```python
from build123d import *

# Parameters (mm, degrees)
SKETCH_1_W      = 6
SKETCH_1_H      = 6
EXTRUDE_1_DEPTH = 3.5
SKETCH_2_R      = 1.75
EXTRUDE_2_DEPTH = 5


with BuildPart() as part:
    # 草图1 → 凸台-拉伸1 (new body)
    with BuildSketch(Plane(origin=(0, 0, 0), x_dir=(1, 0, 0), z_dir=(0, 1, 0))):
        Rectangle(SKETCH_1_W, SKETCH_1_H)
    extrude(amount=EXTRUDE_1_DEPTH)

    # 草图2 → 凸台-拉伸2 (add)
    with BuildSketch(Plane.XZ):
        Circle(SKETCH_2_R)
    extrude(amount=-EXTRUDE_2_DEPTH)


solid = part.part
```
Geometry: final body of the model. Coordinates: model frame, mm. A direction names the side the tool comes from. Coordinates: 2 decimals unless noted, no trailing zeros. Order: outer loops, then holes, each group sorted by start corner. A loop starts at its lowest first (then second) coordinate and runs counter-clockwise, first axis right, second up. Notation, with made-up numbers: (-25, -29) -> (12, -29) arc R8 ccw to (12, -18) -> close; hole circle Ø1 at (-18, -3). An arc over 180 degrees is marked (long way). Use CSV: the item, a comma, the result in double quotes.
1) Section C-C on y = 3.7. Output: boundary loops of the cut face in (x, z), then the cut area to 3 significant figures.
Findings:
outline,"circle Ø3.5 at (0, 0)"
area,"9.62 mm^2"
2) Section A-A on z = 0. Output: boundary loops of the cut face in (x, y), then the cut area to 4 significant figures.
Findings:
outline,"(-3, 0) -> (3, 0) -> (3, 3.5) -> (1.75, 3.5) -> (1.75, 5) -> (-1.75, 5) -> (-1.75, 3.5) -> (-3, 3.5) -> close"
area,"26.25 mm^2"
3) Access query for faces 1 (the flat face through (0, 2, -3)), 2 (the flat face through (1.3, 3.5, -1.4)). Directions: +Z, -Z, +X, -X, +Y, -Y. A direction counts if a zero-diameter tool reaches every point of the face in a straight line with its end or side. Return the directions, or none.
Findings:
face 1,"-Z, +X, -X, +Y, -Y"
face 2,"+Y"
4) Line query: line 1 (Y direction, x = -1.3, z = 2); line 2 (Z direction, x = 1.5, y = 4.05); line 3 (X direction, y = 4, z = -0.35). Output: solid intervals per line, ascending.
Findings:
line 1,"y = 0 to 3.5"
line 2,"z = -0.9 to 0.9"
line 3,"x = -1.71 to 1.71"
5) Section B-B on x = 0. Output: boundary loops of the cut face in (y, z).
Findings:
outline,"(0, -3) -> (3.5, -3) -> (3.5, -1.75) -> (5, -1.75) -> (5, 1.75) -> (3.5, 1.75) -> (3.5, 3) -> (0, 3) -> close"
6) Section D-D on x = -2.3. Output: boundary loops of the cut face in (y, z).
Findings:
outline,"(0, -3) -> (3.5, -3) -> (3.5, 3) -> (0, 3) -> close"
